Verification items for the finished model (mm, model axes). A direction names the side the tool comes from. Round coordinates to 2 decimals unless told otherwise and drop trailing zeros. Order: outer loops, then holes, each group sorted by start corner. A loop starts at its lowest first (then second) coordinate and runs counter-clockwise, first axis right, second up.
```python
from build123d import *

# Parameters (mm, degrees)
BOSS_EXTRUDE2_DEPTH      = 1.5
BOSS_EXTRUDE3_DEPTH      = 5
BOSS_EXTRUDE3_DEPTH_BACK = 5
FILLET1_R                = 1.5


with BuildPart() as part:
    # Sketch1 → Boss-Extrude2 (new body)
    with BuildSketch(Plane.XY):
        Polygon((0, 0), (98, 0), (98, -20), (100, -20), (100, 0), (198, 0), (188, -40), (10, -40), align=None)
    extrude(amount=BOSS_EXTRUDE2_DEPTH)

    # Sketch5 → Boss-Extrude3 (add, two sides)
    with BuildSketch(Plane.XY.offset(1.5)) as boss_extrude3_sk:
        Polygon((186.82883539, -38.5), (196.45383539, 0), (198, 0), (188, -40), (10, -40), (0, 0), (1.54616461, 0), (11.17116461, -38.5), align=None)
    extrude(amount=BOSS_EXTRUDE3_DEPTH)
    extrude(boss_extrude3_sk.sketch, amount=-BOSS_EXTRUDE3_DEPTH_BACK)

    # Fillet1
    fillet1_edges = [part.edges().sort_by_distance(p)[0] for p in [
        (188, -40, 1.5),
        (10, -40, 1.5),
        (191.64133539, -19.25, 0),
        (99, -38.5, 0),
        (6.35866461, -19.25, 0),
        (6.35866461, -19.25, 1.5),
        (99, -38.5, 1.5),
        (191.64133539, -19.25, 1.5),
    ]]
    fillet(fillet1_edges, radius=FILLET1_R)


solid = part.part
```
1) Go/stop test with flat-tipped pins: pin 1 Ø1 at (x, y) = (85, -21.5) entering from +Z; pin 2 Ø1 at (x, z) = (142, -3) entering from +Y; pin 3 Ø3 at (y, z) = (-31.5, 5) entering from -X. Record where each tip stops, or that it passes through.
2) Sectioned sample at A-A on z = 4.5. Record the cut outline in (x, y).
3) Tool access check on faces 1 (the flat face through (6.29, -18.98, -2.49)), 2 (the flat face through (149, 0, 1)), 3 (the cylindrical face through (6.841, -19.416, 1.951)). Record the directions out of +Z, -Z, +X, -X, +Y, -Y that give a thin tool (end or side, any length) a straight path to the whole face; none if there is none.
4) Scan lines: probe 1 along Z at (x, y) = (154.5, -34); probe 2 along Y at (x, z) = (184, 4.5); probe 3 along X at (y, z) = (-6.5, 3.5) (3 decimals). Record each from-to range of solid material in increasing order.
5) Sectioned sample at B-B on x = 56.5. Record the cut outline in (y, z), then the cut area to 3 significant figures.
6) Draft check along X on faces 4 (the flat face through (100, -40, 1)), 5 (the flat face through (5, -20, 2)), 6 (the cylindrical face through (191.29, -18.88, 1.95)). Enter one of: released by +X, released by -X, zero draft, split by the parting line, or undercut.
Returned:
1. pin 1: stops at z = 1.5
1. pin 2: stops at y = -38.5
1. pin 3: stops at x = 7.5
2. outline: (0, 0) - (9.72, -38.86) arc R1.5 ccw to (11.17, -40) - (186.83, -40) arc R1.5 ccw to (188.28, -38.86) - (198, 0) - (196.45, 0) - (186.83, -38.5) - (11.17, -38.5) - (1.55, 0) - close
3. face 1: -Z, +Y
3. face 2: +Z, -Z, +X, -X, +Y
3. face 3: +Z, +Y
4. probe 1: z = 0 to 1.5
4. probe 2: y = -40 to -38.5
4. probe 3: x = 1.625 to 3.171, 194.829 to 196.375
5. outline: (-40, -3.5) - (-38.5, -3.5) - (-38.5, -1.5) arc R1.5 cw to (-37, 0) - (0, 0) - (0, 1.5) - (-37, 1.5) arc R1.5 cw to (-38.5, 3) - (-38.5, 6.5) - (-40, 6.5) - close
5. area: 73.7 mm2
6. face 4: zero draft
6. face 5: released by -X
6. face 6: undercut
